Geometry check sheet. Reference: the model listing, model coordinates, mm. A direction names the side the tool comes from. Give positions to 0.01 mm unless a question says otherwise; leave off trailing zeros. Write each loop counter-clockwise with the first axis right and the second up, starting at its lowest first coordinate (ties: lowest second). Pieces come first, ordered by that corner, then holes. Notation, with made-up numbers: (-23, 23) -> (23, 23) arc R17 cw to (23, 35) -> close; hole circle Ø8 at (-12, 0). An arc over 180 degrees is marked (long way). One line per item, written item: value.
from build123d import *

# Parameters (mm, degrees)
SKETCH1_R           = 7.5
BOSS_EXTRUDE1_DEPTH = 11
SKETCH2_R           = 3
BOSS_EXTRUDE2_DEPTH = 1
SKETCH3_W           = 9
SKETCH3_H           = 12
BOSS_EXTRUDE3_DEPTH = 9
SKETCH4_R           = 2
BOSS_EXTRUDE4_DEPTH = 0.7
SKETCH5_R           = 1.5
BOSS_EXTRUDE5_DEPTH = 10
CUT_EXTRUDE1_DEPTH  = 10
SKETCH7_R           = 0.8
CUT_EXTRUDE2_DEPTH  = 5
SKETCH8_R           = 0.8
CUT_EXTRUDE3_DEPTH  = 5


with BuildPart() as part:
    # Sketch1 → Boss-Extrude1 (new body)
    with BuildSketch(Plane(origin=(0, 0, 0), x_dir=(1, 0, 0), z_dir=(0, 1, 0))):
        with Locations(Location((0, 0, 0), (0, 0, 270))):
            Circle(SKETCH1_R)
    extrude(amount=BOSS_EXTRUDE1_DEPTH)

    # Sketch2 → Boss-Extrude2 (add)
    with BuildSketch(Plane(origin=(0, 11, 0), x_dir=(1, 0, 0), z_dir=(0, 1, 0))):
        with Locations(Location((0, 0, 0), (0, 0, 270))):
            Circle(SKETCH2_R)
    extrude(amount=BOSS_EXTRUDE2_DEPTH)

    # Sketch3 → Boss-Extrude3 (add)
    with BuildSketch(Plane.XZ):
        Rectangle(SKETCH3_W, SKETCH3_H)
    extrude(amount=BOSS_EXTRUDE3_DEPTH)

    # Sketch4 → Boss-Extrude4 (add)
    with BuildSketch(Plane.XZ.offset(9)):
        with Locations(Location((0, 0, 0), (0, 0, 270))):
            Circle(SKETCH4_R)
    extrude(amount=BOSS_EXTRUDE4_DEPTH)

    # Sketch5 → Boss-Extrude5 (add)
    with BuildSketch(Plane.XZ.offset(9.7)):
        with Locations(Location((0, 0, 0), (0, 0, 270))):
            Circle(SKETCH5_R)
    extrude(amount=BOSS_EXTRUDE5_DEPTH)

    # Sketch6 → Cut-Extrude1 (cut)
    with BuildSketch(Plane.XZ.offset(19.7)):
        Polygon((1, 35.32716531), (1, 1.118033989), (1, -1.118033989), (1, -35.32716531), (69.418262642, -35.32716531), (69.418262642, 35.32716531), align=None)
    extrude(amount=-CUT_EXTRUDE1_DEPTH, mode=Mode.SUBTRACT)

    # Sketch7 → Cut-Extrude2 (cut)
    with BuildSketch(Plane.XZ.offset(9)):
        with Locations(Location((0, 4.5, 0), (0, 0, 270))):
            Circle(SKETCH7_R)
        with Locations(Location((0, -4.5, 0), (0, 0, 270))):
            Circle(SKETCH7_R)
    extrude(amount=-CUT_EXTRUDE2_DEPTH, mode=Mode.SUBTRACT)

    # Sketch8 → Cut-Extrude3 (cut)
    with BuildSketch(Plane(origin=(0, 11, 0), x_dir=(1, 0, 0), z_dir=(0, 1, 0))):
        with Locations(Location((0, 4.6, 0), (0, 0, 270))):
            Circle(SKETCH8_R)
        with Locations(Location((0, -4.6, 0), (0, 0, 270))):
            Circle(SKETCH8_R)
    extrude(amount=-CUT_EXTRUDE3_DEPTH, mode=Mode.SUBTRACT)


solid = part.part
1) Mould release check, pull along X, two halves, no side actions. Record for faces 1 (the flat face through (1, -15, 0)), 2 (the cylindrical face through (0, -6.5, -3.7)), 3 (the flat face through (-6, 0, 0)), 4 (the flat face through (0, -4, -4)): released by +X, released by -X, zero draft, split by the parting line, or undercut.
Verdict:
face 1: released by +X
face 2: undercut
face 3: zero draft
face 4: undercut
2) Sectioned sample at B-B on y = -11. Record the cut outline in (x, z), plus the area to 3 significant figures.
Verdict:
outline: (1, -1.12) -> (1, 1.12) arc R1.5 ccw (long way) to start
area: 6.29 mm^2
3) Sectioned sample at D-D on z = -4.5. Record the cut outline in (x, y).
Verdict:
outline: (-6, 0) -> (-4.5, 0) -> (-4.5, -9) -> (-0.8, -9) -> (-0.8, -4) -> (0.8, -4) -> (0.8, -9) -> (4.5, -9) -> (4.5, 0) -> (6, 0) -> (6, 11) -> (0.79, 11) -> (0.79, 6) -> (-0.79, 6) -> (-0.79, 11) -> (-6, 11) -> close
4) Scan lines: probe 1 along Y at (x, z) = (1.5, -4); probe 2 along X at (y, z) = (-6.5, -3.5); probe 3 along Z at (x, y) = (-2.5, -5). Record each from-to range of solid material in increasing order.
Verdict:
probe 1: -9 to 11
probe 2: -4.5 to 4.5
probe 3: -6 to 6
5) Tool access check on faces 5 (the flat face through (6, 0, 0)), 6 (the flat face through (0, 0, -7)), 7 (the flat face through (0.1, 11, 3.2)), 8 (the cylindrical face through (-1.952, -9.345, 0.434)), 9 (the flat face through (0, -4, 6)). Record the directions out of +Z, -Z, +X, -X, +Y, -Y that give a thin tool (end or side, any length) a straight path to the whole face; none if there is none.
Verdict:
face 5: +Z, -Z, +X, -Y
face 6: -Z, +X, -X, -Y
face 7: +Y
face 8: -Y
face 9: +Z, +X, -X, -Y
6) Depth check by flat-ended pin: pin 1 Ø1.8 at (x, z) = (-0.5, -4.5) entering from +Y; pin 2 Ø0.5 at (x, z) = (0.5, 4.5) entering from -Y; pin 3 Ø3.5 at (x, z) = (-5.5, -2.5) entering from -Y. Enter the tip coordinate at first touch or a pass-through.
Verdict:
pin 1: y = 11
pin 2: y = -4
pin 3: y = -9
7) Sectioned sample at C-C on x = -2.5. Record the cut outline in (y, z).
Verdict:
outline: (-9, -6) -> (0, -6) -> (0, -7.07) -> (11, -7.07) -> (11, -1.66) -> (12, -1.66) -> (12, 1.66) -> (11, 1.66) -> (11, 7.07) -> (0, 7.07) -> (0, 6) -> (-9, 6) -> close
8) Sectioned sample at A-A on z = 0. Record the cut outline in (x, y), plus the area to 3 significant figures.
Verdict:
outline: (-7.5, 0) -> (-4.5, 0) -> (-4.5, -9) -> (-2, -9) -> (-2, -9.7) -> (-1.5, -9.7) -> (-1.5, -19.7) -> (1, -19.7) -> (1, -9.7) -> (2, -9.7) -> (2, -9) -> (4.5, -9) -> (4.5, 0) -> (7.5, 0) -> (7.5, 11) -> (3, 11) -> (3, 12) -> (-3, 12) -> (-3, 11) -> (-7.5, 11) -> close
area: 280 mm^2
